```python
from build123d import *

# Parameters (mm, degrees)
F0_R     = 2.75
F1_DEPTH = 3
F2_DEPTH = 6
F3_R     = 2
F4_DEPTH = 25


with BuildPart() as f1:
    # F0 (on Top) → F1 (new body)
    with BuildSketch(Plane.XY):
        Polygon((0, 63), (0, 0), (53, 0), (53, 65), (50, 65), (47.5, 68), (45.2, 68), (17.5, 68), (15.5, 68), (13, 65), (2, 65), align=None)
        with Locations((3, 15)):
            Circle(F0_R, mode=Mode.SUBTRACT)
        with Locations((49.8936027288, 13.5)):
            Circle(F0_R, mode=Mode.SUBTRACT)
        with BuildLine():
            ThreePointArc((20.25, 65.25), (15.5554563517, 63.3054563517), (17.5, 68))
            ThreePointArc((17.5, 68), (19.4445436483, 67.1945436483), (20.25, 65.25))
        make_face(mode=Mode.SUBTRACT)
        with BuildLine():
            ThreePointArc((47.95, 65.25), (43.2554563517, 63.3054563517), (45.2, 68))
            ThreePointArc((45.2, 68), (47.1445436483, 67.1945436483), (47.95, 65.25))
        make_face(mode=Mode.SUBTRACT)
        with BuildLine():
            ThreePointArc((47.95, 65.25), (47.1445436483, 67.1945436483), (45.2, 68))
            ThreePointArc((45.2, 68), (43.2554563517, 63.3054563517), (47.95, 65.25))
        make_face()
        with BuildLine():
            ThreePointArc((20.25, 65.25), (19.4445436483, 67.1945436483), (17.5, 68))
            ThreePointArc((17.5, 68), (15.5554563517, 63.3054563517), (20.25, 65.25))
        make_face()
        with Locations((3, 15)):
            Circle(F0_R)
        with Locations((49.8936027288, 13.5)):
            Circle(F0_R)
    extrude(amount=-F1_DEPTH)

    # F0 (on Top) → F2 (join)
    with BuildSketch(Plane.XY):
        with BuildLine():
            ThreePointArc((20.25, 65.25), (19.4445436483, 67.1945436483), (17.5, 68))
            ThreePointArc((17.5, 68), (15.5554563517, 63.3054563517), (20.25, 65.25))
        make_face()
        with BuildLine():
            ThreePointArc((47.95, 65.25), (47.1445436483, 67.1945436483), (45.2, 68))
            ThreePointArc((45.2, 68), (43.2554563517, 63.3054563517), (47.95, 65.25))
        make_face()
        with Locations((49.8936027288, 13.5)):
            Circle(F0_R)
        with Locations((3, 15)):
            Circle(F0_R)
    extrude(amount=F2_DEPTH)

    # F3 (on face) → F4 (cut)
    with BuildSketch(Plane(origin=(0, 0, -3), x_dir=(1, 0, 0), z_dir=(0, 0, -1))):
        with Locations((42.5, -44)):
            Circle(F3_R)
        with Locations((10.5, -44)):
            Circle(F3_R)
        with Locations((14, -8)):
            Circle(F3_R)
    extrude(amount=-F4_DEPTH, mode=Mode.SUBTRACT)


solid = f1.part
```
CAD build for the part. Positions are in the model's coordinates, mm. A direction names the side the tool comes from. Round coordinates to 2 decimals unless told otherwise and drop trailing zeros. Write each loop counter-clockwise with the first axis right and the second up, starting at its lowest first coordinate (ties: lowest second). Pieces come first, ordered by that corner, then holes. Notation, with made-up numbers: (65, 61.5) - (87, 61.5) arc R22 cw to (87, 89.5) - close; hole circle Ø9 at (9, 44). An arc over 180 degrees is marked (long way). Write item = value, one per line. Start each with the question number.
Q1. Probe L1, parallel to X at y = 44, z = -2.1; L2, parallel to Y at x = 42.5, z = -1.7; L3, parallel to Z at x = 20.5, y = 61. List the from-to ranges inside material, lowest first. Write a range as from..to.
Q2. Band-saw the part on B-B (z = -0.75). Give the cut face in (x, y).
Q3. Band-saw the part on D-D (y = 15). Give the cut face in (x, z), then the cut area to 3 significant figures.
Q4. Drop flat-ended pins along their axis: pin 1 (5 mm diameter, centred on x = 10.5, y = 44, fed in from +Z); pin 2 (2.5 mm diameter, centred on x = 42.5, y = 44, fed in from +Z); pin 3 (1 mm diameter, centred on x = 5.5, z = 3.5, fed in from +Y); pin 4 (1.5 mm diameter, centred on x = 51.5, z = -2, fed in from +Y). Give the stop position or say it passes through.
Q5. Which spindle directions (+Z, -Z, +X, -X, +Y, -Y) get a long thin tool onto all of the face, cutting with end or side? Do faces 4 (the cylindrical face through (2.642, 17.727, 2.958)), 5 (the flat face through (48.768, 66.479, -1.479)). Say none if no direction does.
Q6. Band-saw the part on A-A (y = 44). Give the cut face in (x, z), then the cut area to 3 significant figures.
Q7. Band-saw the part on C-C (x = 14). Give the cut face in (y, z).
Q8. Mould opens along Y. For faces 1 (the flat face through (52, 65, -1)), 2 (the cylindrical face through (10.066, 45.952, -1.521)), 3 (the flat face through (17, 65, 6)) say: pulls with the +Y half, pulls with the -Y half, needs draft (parallel to the pull), parting line crosses it, or undercut.
Answers below:
q1.L1 = 0..8.5, 12.5..40.5, 44.5..53
q1.L2 = 0..42, 46..68
q1.L3 = -3..0
q2.outline = (0, 0) - (53, 0) - (53, 65) - (50, 65) - (47.5, 68) - (15.5, 68) - (13, 65) - (2, 65) - (0, 63) - close; hole circle Ø4 at (10.5, 44); hole circle Ø4 at (14, 8); hole circle Ø4 at (42.5, 44)
q3.outline = (0, -3) - (53, -3) - (53, 0) - (52.2, 0) - (52.2, 6) - (47.59, 6) - (47.59, 0) - (5.75, 0) - (5.75, 6) - (0.25, 6) - (0.25, 0) - (0, 0) - close
q3.area = 220 mm2
q4.pin_1 = 0
q4.pin_2 = through
q4.pin_3 = 16.89
q4.pin_4 = 65
q5.face_4 = +Z
q5.face_5 = +Z, -Z, +X, +Y
q6.outline = (0, -3) - (8.5, -3) - (8.5, 0) - (0, 0) - close; (12.5, -3) - (40.5, -3) - (40.5, 0) - (12.5, 0) - close; (44.5, -3) - (53, -3) - (53, 0) - (44.5, 0) - close
q6.area = 135 mm2
q7.outline = (0, -3) - (6, -3) - (6, 0) - (0, 0) - close; (10, -3) - (66.2, -3) - (66.2, 0) - (10, 0) - close
q8.face_1 = pulls with the +Y half
q8.face_2 = undercut
q8.face_3 = needs draft
